from build123d import *

# Parameters (mm, degrees)
SKETCH_1_R      = 7
EXTRUDE_1_DEPTH = 49
SKETCH_2_R      = 2.5
EXTRUDE_2_DEPTH = 1
FILLET_1_R      = 1


with BuildPart() as part:
    # 草图1 → 凸台-拉伸1 (new body)
    with BuildSketch(Plane(origin=(0, 0, 0), x_dir=(1, 0, 0), z_dir=(0, 1, 0))):
        with Locations(Location((0, 0, 0), (0, 0, 270))):
            Circle(SKETCH_1_R)
    extrude(amount=EXTRUDE_1_DEPTH)

    # 草图2 → 凸台-拉伸2 (add)
    with BuildSketch(Plane(origin=(0, 49, 0), x_dir=(1, 0, 0), z_dir=(0, 1, 0))):
        with Locations(Location((0, 0, 0), (0, 0, 270))):
            Circle(SKETCH_2_R)
    extrude(amount=EXTRUDE_2_DEPTH)

    # 圆角1
    fillet_1_edges = [part.edges().sort_by_distance(p)[0] for p in [
        (0, 0, -7),
        (0, 49, -7),
    ]]
    fillet(fillet_1_edges, radius=FILLET_1_R)


solid = part.part
The listing builds one solid part. Answer for the finished solid, in the listing's coordinates (mm). A direction names the side the tool comes from. Round coordinates to 2 decimals unless told otherwise and drop trailing zeros. Write each loop counter-clockwise with the first axis right and the second up, starting at its lowest first coordinate (ties: lowest second). Pieces come first, ordered by that corner, then holes. Notation, with made-up numbers: M -1.5,55 L 27.5,55 A21 cw 27.5,85 Z; hole C -6,23 d6. An arc over 180 degrees is marked long. Write each question's results on one line, items separated by ' | '. Start each with the question number.
Item 1: Straight lines are drawn through the part: L1, parallel to Y at x = 0.75, z = -3; L2, parallel to Z at x = -1, y = 6; L3, parallel to Z at x = 3.5, y = 20.5. For each, find the intervals that lie inside material, in ascending order. Write a range as [from, to].
Item 2: Flat-ended cylindrical pins translate along their axes: pin 1 Ø1.5 at (x, y) = (-5.5, 14) entering from -Z; pin 2 Ø1.5 at (y, z) = (36, 2) entering from -X; pin 3 Ø4 at (y, z) = (6, 3) entering from +X. Find the tip coordinate at first contact, or state that the pin passes through.
Item 3: A cutting plane is placed at A-A on y = 17. Write down the section's boundary in (x, z).
Item 4: For faces 1 (the face through (0, 49, 3)), 2 (the face through (0, 0, 0)), determine the directions among +Z, -Z, +X, -X, +Y, -Y from which every point of the face is accessible in a straight line to the end or side of a thin tool.
Check sheet entries:
1) L1: [0, 49] | L2: [-6.93, 6.93] | L3: [-6.06, 6.06]
2) pin 1: z = -5.14 | pin 2: x = -6.89 | pin 3: x = 6.93
3) outline: C 0,0 d14
4) face 1: +Y | face 2: +Z, -Z, +X, -X, -Y
